```python
from build123d import *

# Parameters (mm, degrees)
SKETCH_1_W          = 15
SKETCH_1_H          = 20
EXTRUDE_1_DEPTH     = 10
SKETCH_2_W          = 15
SKETCH_2_H          = 20
SKETCH_2_R          = 2
EXTRUDE_2_DEPTH     = 20
SKETCH_3_W          = 20
SKETCH_3_H          = 10
CUT_EXTRUDE_1_DEPTH = 33.015621187
FILLET_1_RADIUS     = 7.5
FILLET_1_LENGTH     = 5
FILLET_2_RADIUS     = 7.5
FILLET_2_LENGTH     = 5
SKETCH_4_R          = 1.5
CUT_EXTRUDE_2_DEPTH = 40.05124838


with BuildPart() as part:
    # 草图1 → 凸台-拉伸1 (new body)
    with BuildSketch(Plane.XY):
        with Locations((7.5, 10)):
            Rectangle(SKETCH_1_W, SKETCH_1_H)
    extrude(amount=EXTRUDE_1_DEPTH)

    # 草图2 → 凸台-拉伸2 (add)
    with BuildSketch(Plane.XZ):
        with Locations((7.5, -10)):
            Rectangle(SKETCH_2_W, SKETCH_2_H)
        with Locations(Location((7.5, -11, 0), (0, 0, 270))):
            Circle(SKETCH_2_R, mode=Mode.SUBTRACT)
    extrude(amount=-EXTRUDE_2_DEPTH)

    # 草图3 → 切除-拉伸1 (cut, through all)
    with BuildSketch(Plane(origin=(15, 0, 0), x_dir=(0, 0, -1), z_dir=(1, 0, 0))):
        with Locations((10, 10)):
            Rectangle(SKETCH_3_W, SKETCH_3_H)
    extrude(amount=-CUT_EXTRUDE_1_DEPTH, mode=Mode.SUBTRACT)

    # 圆角1: full round fillet: the end face becomes a half cylinder, R = half its width
    fillet_1_face = Plane((7.5, 17.5, -20), x_dir=(0, 1, 0), z_dir=(0, 0, -1))  # on the end face: x along it, z out of the body
    fillet_1_slab = fillet_1_face.offset(-FILLET_1_RADIUS / 2) * Box(FILLET_1_LENGTH, 2 * FILLET_1_RADIUS, FILLET_1_RADIUS, mode=Mode.PRIVATE)  # the body's end, R deep
    fillet_1_round = Plane((7.5, 17.5, -12.5), x_dir=(0, 0, -1), z_dir=(0, 1, 0)) * Cylinder(FILLET_1_RADIUS, FILLET_1_LENGTH, mode=Mode.PRIVATE)  # its axis R under the face
    add(fillet_1_slab - fillet_1_round, mode=Mode.SUBTRACT)

    # 圆角2: full round fillet: the end face becomes a half cylinder, R = half its width
    fillet_2_face = Plane((7.5, 2.5, -20), x_dir=(0, -1, 0), z_dir=(0, 0, -1))  # on the end face: x along it, z out of the body
    fillet_2_slab = fillet_2_face.offset(-FILLET_2_RADIUS / 2) * Box(FILLET_2_LENGTH, 2 * FILLET_2_RADIUS, FILLET_2_RADIUS, mode=Mode.PRIVATE)  # the body's end, R deep
    fillet_2_round = Plane((7.5, 2.5, -12.5), x_dir=(0, 0, -1), z_dir=(0, -1, 0)) * Cylinder(FILLET_2_RADIUS, FILLET_2_LENGTH, mode=Mode.PRIVATE)  # its axis R under the face
    add(fillet_2_slab - fillet_2_round, mode=Mode.SUBTRACT)

    # 草图4 → 切除-拉伸2 (cut, through all)
    with BuildSketch(Plane.XY.offset(10)):
        with Locations((10, 10)):
            Circle(SKETCH_4_R)
    extrude(amount=-CUT_EXTRUDE_2_DEPTH, mode=Mode.SUBTRACT)


solid = part.part
```
Verification items for the finished model (mm, model axes). A direction names the side the tool comes from. Give positions to 0.01 mm unless a question says otherwise; leave off trailing zeros. Order: outer loops, then holes, each group sorted by start corner. A loop starts at its lowest first (then second) coordinate and runs counter-clockwise, first axis right, second up. Notation, with made-up numbers: M 52.5,50.5 L 72.5,50.5 A18 cw 72.5,63.5 Z; hole C 32,26.25 d8. An arc over 180 degrees is marked long. Answer in a Markdown table with one row per item. Add a question column.
Item 1: Scan lines: probe 1 along Y at (x, z) = (5, -11); probe 2 along Y at (x, z) = (10, 2.5); probe 3 along X at (y, z) = (18.9, -11). Record each from-to range of solid material in increasing order. Write a range as from..to.
Item 2: Mould release check, pull along Z, two halves, no side actions. Record for faces 1 (the cylindrical face through (8.852, 2.465, -9.526)), 2 (the flat face through (8, 5, -8)), 3 (the cylindrical face through (7.66, 17.54, -20)): released by +Z, released by -Z, zero draft, split by the parting line, or undercut.
Item 3: Tool access check on faces 4 (the flat face through (8, 10, 0)), 5 (the flat face through (7, 10, 10)). Record the directions out of +Z, -Z, +X, -X, +Y, -Y that give a thin tool (end or side, any length) a straight path to the whole face; none if there is none.
Item 4: Section check D-D, the plane z = -3.75. Enter the section's corners in (x, y).
Item 5: Section check A-A, the plane y = 10. Enter the section's corners in (x, z).
Item 6: Gauge pin test, flat ends, axial feed: pin 1 (8 mm diameter, centred on x = 10.5, y = 8, fed in from -Z); pin 2 (8 mm diameter, centred on x = 5.5, z = -9.5, fed in from -Y). Record the tip position at first contact, or that the pin passes through.
Item 7: Section check B-B, the plane z = -11. Enter the section's corners in (x, y), and give its area (3 significant figures).
Item 8: Section check C-C, the plane x = 7.5. Enter the section's corners in (y, z).
Filled sheet:
| question | item | result |
|---|---|---|
| 1 | probe 1 | y = 0..5, 15..20 |
| 1 | probe 2 | y = 0..8.5, 11.5..20 |
| 1 | probe 3 | x = 0..5.5, 9.5..15 |
| 2 | face 1 | undercut |
| 2 | face 2 | zero draft |
| 2 | face 3 | released by -Z |
| 3 | face 4 | -Z, +X, -X |
| 3 | face 5 | +Z, +X, -X, +Y, -Y |
| 4 | outline | M 0,0 L 15,0 L 15,5 L 0,5 Z; M 0,15 L 15,15 L 15,20 L 0,20 Z |
| 5 | outline | M 0,0 L 8.5,0 L 8.5,10 L 0,10 Z; M 11.5,0 L 15,0 L 15,10 L 11.5,10 Z |
| 6 | pin 1 | stops at z = -19.99 |
| 6 | pin 2 | stops at y = 0 |
| 7 | outline | M 0,0 L 5.5,0 L 5.5,5 L 0,5 Z; M 0,15 L 5.5,15 L 5.5,20 L 0,20 Z; M 9.5,0 L 15,0 L 15,5 L 9.5,5 Z; M 9.5,15 L 15,15 L 15,20 L 9.5,20 Z |
| 7 | area | 110 mm^2 |
| 8 | outline | M 0,-20 L 5,-20 L 5,-13 L 0,-13 Z; M 0,-9 L 5,-9 L 5,0 L 15,0 L 15,-9 L 20,-9 L 20,10 L 0,10 Z; M 15,-20 L 20,-20 L 20,-13 L 15,-13 Z |
